The listing builds one solid part. Answer for the finished solid, in the listing's coordinates (mm). A direction names the side the tool comes from. Round coordinates to 2 decimals unless told otherwise and drop trailing zeros. Write each loop counter-clockwise with the first axis right and the second up, starting at its lowest first coordinate (ties: lowest second). Pieces come first, ordered by that corner, then holes. Notation, with made-up numbers: (-19, -26.5) - (19, -26.5) arc R10 cw to (19, -19.5) - close; hole circle Ø4 at (24.25, 13). An arc over 180 degrees is marked (long way). Answer in a Markdown table with one row per item.
from build123d import *

# Parameters (mm, degrees)
SKETCH1_W               = 95.25
SKETCH1_H               = 95.25
BOSS_EXTRUDE1_DEPTH     = 57.15
SHELL1_T                = -3.81
SKETCH2_R               = 3.048
BOSS_EXTRUDE2_DEPTH     = 22.86
BOSS_EXTRUDE3_START     = -24.13
SKETCH5_R               = 3.048
BOSS_EXTRUDE3_DEPTH     = 22.86
SKETCH6_W               = 11.999999876
SKETCH6_H               = 4.800000052
CUT_EXTRUDE1_DEPTH      = 3.81
BOSS_EXTRUDE4_DEPTH     = 19.812
SKETCH9_W               = 95.25
SKETCH9_H               = 3.81
BOSS_EXTRUDE5_DEPTH     = 95.25
SKETCH10_W              = 87.63
SKETCH10_H              = 8.89
CUT_EXTRUDE2_DEPTH      = 23.622
SKETCH11_W              = 87.63
SKETCH11_H              = 8.89
CUT_EXTRUDE3_DEPTH      = 23.622
FILLET1_R               = 2.54
BOSS_EXTRUDE6_START     = -47.625
BOSS_EXTRUDE6_DEPTH     = 22.225
CUT_EXTRUDE4_DEPTH      = 1
CUT_EXTRUDE4_DEPTH_BACK = 3.81


with BuildPart() as part:
    # Sketch1 → Boss-Extrude1 (new body)
    with BuildSketch(Plane(origin=(0, 0, 0), x_dir=(1, 0, 0), z_dir=(0, 1, 0))):
        Rectangle(SKETCH1_W, SKETCH1_H)
    extrude(amount=BOSS_EXTRUDE1_DEPTH)

    # Shell1
    shell1_openings = [part.faces().sort_by_distance(p)[0] for p in [
        (0, 57.15, 0),
    ]]
    offset(amount=SHELL1_T, openings=shell1_openings, kind=Kind.INTERSECTION)

    # Sketch2 → Boss-Extrude2 (add)
    with BuildSketch(Plane.ZY.offset(47.625)):
        with BuildLine():
            ThreePointArc((-50.165, 57.15), (-57.189031836, 61.843308025), (-58.837102448, 53.557897552))
            Line((-58.837102448, 53.557897552), (-47.625, 42.345795103))
            Line((-47.625, 42.345795103), (-47.625, 57.15))
            Line((-47.625, 57.15), (-50.165, 57.15))
        make_face()
        with Locations((-55.245, 57.15)):
            Circle(SKETCH2_R, mode=Mode.SUBTRACT)
    extrude(amount=-BOSS_EXTRUDE2_DEPTH)

    # Sketch5 → Boss-Extrude3 (add)
    with BuildSketch(Plane(origin=(47.625, 0, 0), x_dir=(0, 0, -1), z_dir=(1, 0, 0)).offset(BOSS_EXTRUDE3_START)):
        with BuildLine():
            Line((50.165, 57.15), (47.625, 57.15))
            Line((47.625, 57.15), (47.625, 42.345795103))
            Line((47.625, 42.345795103), (58.837102448, 53.557897552))
            ThreePointArc((58.837102448, 53.557897552), (57.189031836, 61.843308025), (50.165, 57.15))
        make_face()
        with Locations((55.245, 57.15)):
            Circle(SKETCH5_R, mode=Mode.SUBTRACT)
    extrude(amount=-BOSS_EXTRUDE3_DEPTH)

    # Sketch6 → Cut-Extrude1 (cut)
    with BuildSketch(Plane.XY.offset(47.625)):
        with Locations((0, 47.129999974)):
            Rectangle(SKETCH6_W, SKETCH6_H)
    extrude(amount=-CUT_EXTRUDE1_DEPTH, mode=Mode.SUBTRACT)

    # Sketch8 → Boss-Extrude4 (add)
    with BuildSketch(Plane.XZ):
        Polygon((41.275, -42.545), (-42.545, -42.545), (-42.545, 18.415), (41.275, 18.415), (47.625, 18.415), (47.625, 47.625), (-47.625, 47.625), (-47.625, -47.625), (47.625, -47.625), (47.625, -42.545), align=None)
    extrude(amount=BOSS_EXTRUDE4_DEPTH)

    # Sketch9 → Boss-Extrude5 (add, through all)
    with BuildSketch(Plane(origin=(47.625, 0, 0), x_dir=(0, 0, -1), z_dir=(1, 0, 0))):
        with Locations((0, -21.717)):
            Rectangle(SKETCH9_W, SKETCH9_H)
    extrude(amount=-BOSS_EXTRUDE5_DEPTH)

    # Sketch10 → Cut-Extrude2 (cut)
    with BuildSketch(Plane(origin=(0, 3.81, 0), x_dir=(1, 0, 0), z_dir=(0, 1, 0))):
        with Locations((0, 39.37)):
            Rectangle(SKETCH10_W, SKETCH10_H)
    extrude(amount=-CUT_EXTRUDE2_DEPTH, mode=Mode.SUBTRACT)

    # Sketch11 → Cut-Extrude3 (cut)
    with BuildSketch(Plane(origin=(0, 3.81, 0), x_dir=(1, 0, 0), z_dir=(0, 1, 0))):
        with Locations((0, -13.97)):
            Rectangle(SKETCH11_W, SKETCH11_H)
    extrude(amount=-CUT_EXTRUDE3_DEPTH, mode=Mode.SUBTRACT)

    # Fillet1
    fillet1_edges = [part.edges().sort_by_distance(p)[0] for p in [
        (-47.625, 9.361897552, -47.625),
        (47.625, 16.764, -47.625),
        (47.625, 16.764, 47.625),
        (-47.625, 16.764, 47.625),
    ]]
    fillet(fillet1_edges, radius=FILLET1_R)

    # Sketch12 → Boss-Extrude6 (add, symmetric)
    with BuildSketch(Plane(origin=(47.625, 0, 0), x_dir=(0, 0, -1), z_dir=(1, 0, 0)).offset(BOSS_EXTRUDE6_START)):
        Polygon((-47.625, 55.245), (-47.625, 59.055), (-49.911, 60.325), (-49.911, 53.975), align=None)
    extrude(amount=BOSS_EXTRUDE6_DEPTH, both=True)

    # Sketch13 → Cut-Extrude4 (cut, two sides)
    with BuildSketch(Plane.XY.offset(49.911)) as cut_extrude4_sk:
        Polygon((-245.795957614, 57.15), (-22.225, 57.15), (-6.985, 57.15), (-6.985, 60.325), (-6.985, 283.895957614), (-314.864920178, 608.157961407), (-553.675877792, 381.412003793), align=None)
    extrude(amount=CUT_EXTRUDE4_DEPTH, mode=Mode.SUBTRACT)
    extrude(cut_extrude4_sk.sketch, amount=-CUT_EXTRUDE4_DEPTH_BACK, mode=Mode.SUBTRACT)


solid = part.part
(1) Section D-D (z = -32.5) is taken. Give the vertices of the cut face in (x, y) (3 decimals).
Checked values:
| item | result |
|---|---|
| outline | (-47.625, -23.622) - (47.625, -23.622) - (47.625, -19.812) - (-42.545, -19.812) - (-42.545, 0) - (47.625, 0) - (47.625, 57.15) - (43.815, 57.15) - (43.815, 3.81) - (-43.815, 3.81) - (-43.815, 57.15) - (-47.625, 57.15) - close |
(2) For faces 4 (the flat face through (43.815, 27, 1)), 5 (the flat face through (0, 44.73, 46)), 6 (the flat face through (46, -10, -42.545)), determine the directions among +Z, -Z, +X, -X, +Y, -Y from which every point of the face is accessible in a straight line to the end or side of a thin tool.
Checked values:
| item | result |
|---|---|
| face 4 | +Y |
| face 5 | +Z |
| face 6 | +X |
(3) Section C-C (y = 8.5) is taken. Give the vertices of the cut face in (x, z) (3 decimals), and give its area (3 significant figures).
Checked values:
| item | result |
|---|---|
| outline | (-47.625, -45.085) arc R2.54 ccw to (-45.085, -47.625) - (45.085, -47.625) arc R2.54 ccw to (47.625, -45.085) - (47.625, 45.085) arc R2.54 ccw to (45.085, 47.625) - (-45.085, 47.625) arc R2.54 ccw to (-47.625, 45.085) - close; hole (-43.815, -43.815) - (43.815, -43.815) - (43.815, 43.815) - (-43.815, 43.815) - close |
| area | 1,390 mm2 |
(4) For a pull along X with two mould halves and no side action, classify faces 1 (the flat face through (0, 3, -34.925)), 2 (the cylindrical face through (-46.86, 16.2, 46.9)), 3 (the cylindrical face through (12.225, 61.788, -57.317)) as pulls with the +X half, pulls with the -X half, needs draft (parallel to the pull), parting line crosses it, or undercut.
Checked values:
| item | result |
|---|---|
| face 1 | undercut |
| face 2 | pulls with the -X half |
| face 3 | needs draft |
(5) Section A-A (x = -38.5) is taken. Give the vertices of the cut face in (y, z) (3 decimals).
Checked values:
| item | result |
|---|---|
| outline | (-23.622, -47.625) - (42.346, -47.625) - (53.558, -58.837) arc R5.08 ccw (long way) to (57.15, -50.165) - (57.15, -43.815) - (-19.812, -43.815) - (-19.812, 18.415) - (3.81, 18.415) - (3.81, 43.815) - (57.15, 43.815) - (57.15, 47.625) - (-23.622, 47.625) - close; (0, -34.925) - (3.81, -34.925) - (3.81, 9.525) - (0, 9.525) - close; hole circle Ø6.096 at (57.15, -55.245) |
(6) Flat-ended cylindrical pins translate along their axes: pin 1 (4 mm diameter, centred on x = 1, z = 46, fed in from +Y); pin 2 (12 mm diameter, centred on x = -20.5, z = 28, fed in from +Y); pin 3 (1.5 mm diameter, centred on x = 4, y = 58, fed in from -Z); pin 4 (1.8 mm diameter, centred on y = 58.5, z = 48.5, fed in from -X) (3 decimals). Find the tip coordinate at first contact, or state that the pin passes through.
Checked values:
| item | result |
|---|---|
| pin 1 | stops at y = 59.26 |
| pin 2 | stops at y = 3.81 |
| pin 3 | stops at z = -60.32 |
| pin 4 | stops at x = -6.985 |
(7) Find the intervals of material crossed by line 1 (Z direction, x = -38, y = 57) (3 decimals); line 2 (X direction, y = 39, z = -34) (3 decimals); line 3 (Y direction, x = -33.5, z = -5), in increasing order.
Checked values:
| item | result |
|---|---|
| line 1 | z = -60.323 to -58.289, -52.201 to -43.815, 43.815 to 47.625 |
| line 2 | x = -47.625 to -43.815, 43.815 to 47.625 |
| line 3 | y = -23.62 to -19.81, 0 to 3.81 |
(8) Section B-B (x = 38) is taken. Give the vertices of the cut face in (y, z) (3 decimals).
Checked values:
| item | result |
|---|---|
| outline | (-23.622, -47.625) - (57.15, -47.625) - (57.15, -43.815) - (-19.812, -43.815) - (-19.812, 18.415) - (3.81, 18.415) - (3.81, 43.815) - (57.15, 43.815) - (57.15, 47.625) - (-23.622, 47.625) - close; (0, -34.925) - (3.81, -34.925) - (3.81, 9.525) - (0, 9.525) - close |
